Could you check a few things on this model? Use its own coordinates, in mm. Round coordinates to 2 decimals unless told otherwise and drop trailing zeros. Write each loop counter-clockwise with the first axis right and the second up, starting at its lowest first coordinate (ties: lowest second). Pieces come first, ordered by that corner, then holes. Notation, with made-up numbers: (20, 30) -> (76, 30) arc R22 cw to (76, 52) -> close; hole circle Ø7 at (6, 58). An arc over 180 degrees is marked (long way). One line per question, with ' | ' between items. Start each with the question number.
1. Imagine slicing it at A-A, the plane x = 0. List the corners of the cut face in (y, z) for me, and give its area (3 significant figures).
2. Imagine slicing it at D-D, the plane z = -21. List the corners of the cut face in (x, y) for me, and give its area (3 significant figures).
3. Imagine slicing it at B-B, the plane z = 0. List the corners of the cut face in (x, y) for me, and give its area (3 significant figures).
4. If I drill on line 1 along Z through (x, y) = (-49, 1.6); line 2 along X through (y, z) = (4.4, -50); line 3 along Z through (x, y) = (7.5, 3.95), over which ranges is the centre line in solid material (lowest first)? Write a range as [from, to].
5. For pin 1 Ø1 at (x, z) = (-41, 19) entering from -Y; pin 2 Ø1 at (x, y) = (-21, 4.5) entering from +Z; pin 3 Ø1 at (x, z) = (26.5, 11) entering from -Y; pin 4 Ø1.5 at (y, z) = (1.5, 15) entering from -X, each with a flat end and sliding along its axis, tell me the tip position at first contact or that it passes through.
6. Imagine slicing it at C-C, the plane y = 4. State how many separate pieces and enclosed holes the cut face has, and give its area (3 significant figures).
from build123d import *

# Parameters (mm, degrees)
SKETCH1_R           = 60
SKETCH1_R_2         = 2.5
BOSS_EXTRUDE1_DEPTH = 5
SKETCH4_R           = 1.15
CUT_EXTRUDE1_DEPTH  = 5
SKETCH5_W           = 5
SKETCH5_H           = 15
CUT_EXTRUDE2_DEPTH  = 5
SKETCH6_W           = 5
SKETCH6_H           = 15
CUT_EXTRUDE3_DEPTH  = 5


with BuildPart() as part:
    # Sketch1 → Boss-Extrude1 (new body)
    with BuildSketch(Plane(origin=(0, 0, 0), x_dir=(1, 0, 0), z_dir=(0, 1, 0))):
        with Locations(Location((0, 0, 0), (0, 0, 270))):
            Circle(SKETCH1_R)
        with Locations(Location((0, 0, 0), (0, 0, 270))):
            Circle(SKETCH1_R_2, mode=Mode.SUBTRACT)
    extrude(amount=BOSS_EXTRUDE1_DEPTH)

    # Sketch4 → Cut-Extrude1 (cut)
    with BuildSketch(Plane(origin=(0, 5, 0), x_dir=(1, 0, 0), z_dir=(0, 1, 0))):
        with Locations(Location((-6.75, 50, 0), (0, 0, 270))):
            Circle(SKETCH4_R)
        with Locations(Location((50, 6.75, 0), (0, 0, 270))):
            Circle(SKETCH4_R)
        with Locations(Location((6.75, -50, 0), (0, 0, 270))):
            Circle(SKETCH4_R)
        with Locations(Location((-50, -6.75, 0), (0, 0, 270))):
            Circle(SKETCH4_R)
        with Locations(Location((6.75, 50, 0), (0, 0, 90))):
            Circle(SKETCH4_R)
        with Locations(Location((50, -6.75, 0), (0, 0, 90))):
            Circle(SKETCH4_R)
        with Locations(Location((-6.75, -50, 0), (0, 0, 90))):
            Circle(SKETCH4_R)
        with Locations(Location((-50, 6.75, 0), (0, 0, 90))):
            Circle(SKETCH4_R)
    extrude(amount=-CUT_EXTRUDE1_DEPTH, mode=Mode.SUBTRACT)

    # Sketch5 → Cut-Extrude2 (cut)
    with BuildSketch(Plane(origin=(0, 5, 0), x_dir=(1, 0, 0), z_dir=(0, 1, 0))):
        with Locations((-17.5, 17.5)):
            Rectangle(SKETCH5_W, SKETCH5_H)
        with Locations((-17.5, -17.5)):
            Rectangle(SKETCH5_W, SKETCH5_H)
    extrude(amount=-CUT_EXTRUDE2_DEPTH, mode=Mode.SUBTRACT)

    # Sketch6 → Cut-Extrude3 (cut)
    with BuildSketch(Plane(origin=(0, 5, 0), x_dir=(1, 0, 0), z_dir=(0, 1, 0))):
        with Locations((27.5, 17.5)):
            Rectangle(SKETCH6_W, SKETCH6_H)
        with Locations((27.5, -17.5)):
            Rectangle(SKETCH6_W, SKETCH6_H)
    extrude(amount=-CUT_EXTRUDE3_DEPTH, mode=Mode.SUBTRACT)


solid = part.part
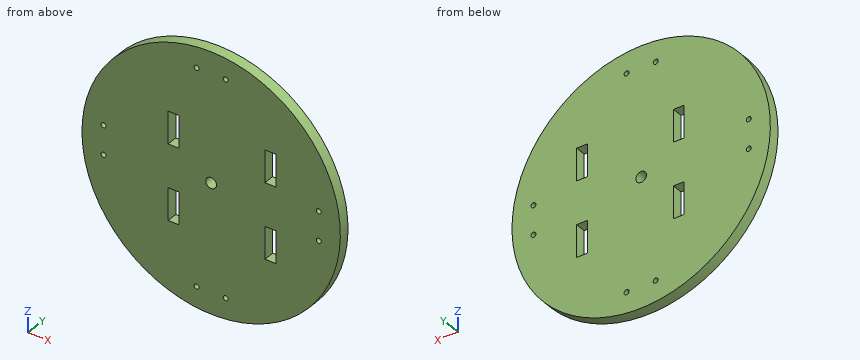
Geometry results:
1) outline: (0, -60) -> (5, -60) -> (5, -2.5) -> (0, -2.5) -> close; (0, 2.5) -> (5, 2.5) -> (5, 60) -> (0, 60) -> close | area: 575 mm2
2) outline: (-56.2, 0) -> (-20, 0) -> (-20, 5) -> (-56.2, 5) -> close; (-15, 0) -> (25, 0) -> (25, 5) -> (-15, 5) -> close; (30, 0) -> (56.2, 0) -> (56.2, 5) -> (30, 5) -> close | area: 512 mm2
3) outline: (-60, 0) -> (-2.5, 0) -> (-2.5, 5) -> (-60, 5) -> close; (2.5, 0) -> (60, 0) -> (60, 5) -> (2.5, 5) -> close | area: 575 mm2
4) line 1: z = [-34.63, -7.32], [-6.18, 6.18], [7.32, 34.63] | line 2: x = [-33.17, -7.9], [-5.6, 5.6], [7.9, 33.17] | line 3: z = [-59.53, -50.87], [-49.13, 49.13], [50.87, 59.53]
5) pin 1: stops at y = 0 | pin 2: stops at z = 56.39 | pin 3: passes through | pin 4: stops at x = -58.28
6) separate pieces: 1 | enclosed holes: 13 | area: 11,000 mm2
